Autodesk Inventor part; units mm, degrees
ref_plane "YZ Plane" through (0, 0, 0) normal (1, 0, 0) x (0, 1, 0)
ref_plane "XZ Plane" through (0, 0, 0) normal (0, 1, 0) x (-1, 0, 0)
ref_plane "XY Plane" through (0, 0, 0) normal (0, 0, 1) x (1, 0, 0)
sketch "Sketch1" plane through (0, 0, 0) normal (0, 1, 0) x (-1, 0, 0)
  circle A0 centre (0, 0) radius 2
  circle A1 centre (0, 0) radius 3
  circle A2 centre (0, 0) radius 4
  dimension "d0" = 4
  dimension "d1" = 6
  dimension "d2" = 8
extrude "Extrusion1" add sketch "Sketch1" along normal blind 0.2 contours A1 | A2
extrude "Extrusion2" add sketch "Sketch1" along normal blind 3.7 contours A1
fillet "Fillet1" radius 2 1 edges at (3, 0.2, 0)
properties part number "replacement standoff"
Here's how the part is built. I have some questions about the finished solid (model axes, mm). Coordinates: 2 decimals unless noted, no trailing zeros. Write each loop counter-clockwise with the first axis right and the second up, starting at its lowest first coordinate (ties: lowest second). Pieces come first, ordered by that corner, then holes. Notation, with made-up numbers: (76, 70.5) - (122, 70.5) arc R14 ccw to (122, 92.5) - close; hole circle Ø3 at (22, 10.25). An arc over 180 degrees is marked (long way). One line per item, written item: value.
1) Suppose I cut it at D-D on y = 0.65. Write out the boundary of the cut face in (x, z), and give its area (3 significant figures).
Model answer:
outline: circle Ø6.93 at (0, 0); hole circle Ø4 at (0, 0)
area: 25.2 mm²
2) Suppose I cut it at B-B on z = 0. Write out the boundary of the cut face in (x, y).
Model answer:
outline: (-4, 0) - (-2, 0) - (-2, 3.7) - (-3, 3.7) - (-3, 1.93) arc R2 cw to (-4, 0.2) - close; (2, 0) - (4, 0) - (4, 0.2) arc R2 cw to (3, 1.93) - (3, 3.7) - (2, 3.7) - close
3) Suppose I cut it at A-A on x = 0. Write out the boundary of the cut face in (y, z).
Model answer:
outline: (0, -4) - (0.2, -4) arc R2 cw to (1.93, -3) - (3.7, -3) - (3.7, -2) - (0, -2) - close; (0, 2) - (3.7, 2) - (3.7, 3) - (1.93, 3) arc R2 cw to (0.2, 4) - (0, 4) - close
4) We'd pull the mould along Z, two halves only. Please class faces 1 (the flat face through (-1, 3.7, -2)), 2 (the cylindrical face through (0, 2, 2)), 3 (the cylindrical face through (3, 3, 0)): pulls with the +Z half, pulls with the -Z half, needs draft (parallel to the pull), parting line crosses it, or undercut.
Model answer:
face 1: needs draft
face 2: undercut
face 3: parting line crosses it
5) I'm going to push flat-ended pins straight in: P1, Ø2, axis at y = 3, z = 0, coming from the +X side; P2, Ø1.5, axis at x = -0.5, y = 1, coming from the +Z side. Where does each tip first touch, or does it pass through?
Model answer:
P1: stops at x = 3
P2: stops at z = 3.89
6) I need wall thicknesses on line 1 along Z through (x, y) = (0, 1.9); line 2 along X through (y, z) = (2.45, 1); line 3 along X through (y, z) = (0.25, -0.25). Which ranges of each line are inside material? Lowest first, please.
Model answer:
line 1: z = -3 to -2, 2 to 3
line 2: x = -2.83 to -1.73, 1.73 to 2.83
line 3: x = -3.91 to -1.98, 1.98 to 3.91
7) Suppose I cut it at C-C on y = 2.35. Write out the boundary of the cut face in (x, z).
Model answer:
outline: circle Ø6 at (0, 0); hole circle Ø4 at (0, 0)
